Autodesk Inventor part; units mm, degrees
ref_plane "YZ Plane" through (0, 0, 0) normal (1, 0, 0) x (0, 1, 0)
ref_plane "XZ Plane" through (0, 0, 0) normal (0, 1, 0) x (-1, 0, 0)
ref_plane "XY Plane" through (0, 0, 0) normal (0, 0, 1) x (1, 0, 0)
sketch "Skizze1" plane through (0, 0, 0) normal (0, 0, 1) x (1, 0, 0)
  line L0 (0, 370.86) -> (0, -370.86)
  line L1 (-560, 0) -> (560, 0)
  line L2 (400, -264.9) -> (-400, -264.9)
  line L3 (-400, -264.9) -> (-400, 264.9)
  line L4 (-400, 264.9) -> (400, 264.9)
  line L5 (400, 264.9) -> (400, -264.9)
  point P0 (0, 0)
  point P1 (0, -264.9)
  point P2 (-400, 0)
  dimension "d0" = 800
  dimension "d1" = 529.8
extrude "Extrusion1" add sketch "Skizze1" along normal blind 4
sketch "Skizze2" plane through (0, 0, 0) normal (0, 0, -1) x (-1, 0, 0)
  line L0 (400, 264.9) -> (400, -264.9)
  line L1 (-400, 264.9) -> (400, 264.9)
  point P0 (0, 0)
  point P1 (350, 50)
  point P2 (350, 0)
  point P3 (350, -50)
  dimension "d4" = 50
  dimension "d5" = 50
  dimension "d6" = 50
  dimension "d7" = 50
  dimension "d8" = 50
  dimension "d9" = 264.9
hole "Bohrung1" at (-350, 50, 0) at (-350, 0, 0) at (-350, -50, 0) direction (0, 0, 1) diameter 40 end through all
properties part number "Käfigboden" material "PVC-U"
Build history of the part. All positions in model axes, mm. Coordinates: 2 decimals unless noted, no trailing zeros. Write each loop counter-clockwise with the first axis right and the second up, starting at its lowest first coordinate (ties: lowest second). Pieces come first, ordered by that corner, then holes.
1. Drop a flat-ended pin along its axis: pin 1 (24 mm diameter, centred on x = -350, y = 0, fed in from -Z). Give the stop position or say it passes through.
Answer block:
pin 1: passes through
2. Pull direction Y, two halves, no side cores. Call faces 1 (the cylindrical face through (-330.476, -54.336, 2.028)), 2 (the flat face through (-6, 4, 4)): released by +Y, released by -Y, zero draft, split by the parting line, or undercut.
Answer block:
face 1: undercut
face 2: zero draft
3. Band-saw the part on A-A, the plane x = -350. Give the cut face in (y, z).
Answer block:
outline: (-264.9, 0) - (-70, 0) - (-70, 4) - (-264.9, 4) - close; (-30, 0) - (-20, 0) - (-20, 4) - (-30, 4) - close; (20, 0) - (30, 0) - (30, 4) - (20, 4) - close; (70, 0) - (264.9, 0) - (264.9, 4) - (70, 4) - close
4. Drill centre lines: probe 1 along Y at (x, z) = (-350, 1.75); probe 2 along X at (y, z) = (-50, 2.25); probe 3 along X at (y, z) = (-42, 2.7). Where is each one in solid material? Low to high.
Answer block:
probe 1: y = -264.9 to -70, -30 to -20, 20 to 30, 70 to 264.9
probe 2: x = -400 to -370, -330 to 400
probe 3: x = -400 to -368.33, -331.67 to 400
5. Band-saw the part on B-B, the plane y = 50. Give the cut face in (x, z), and give its area (3 significant figures).
Answer block:
outline: (-400, 0) - (-370, 0) - (-370, 4) - (-400, 4) - close; (-330, 0) - (400, 0) - (400, 4) - (-330, 4) - close
area: 3,040 mm2
